Input: part model. Units: mm. Frame: model coordinates. A direction names the side the tool comes from. Coordinates: 2 decimals unless noted, no trailing zeros. Order: outer loops, then holes, each group sorted by start corner. A loop starts at its lowest first (then second) coordinate and runs counter-clockwise, first axis right, second up. Notation, with made-up numbers: (-17, -16) -> (4, -16) arc R20 ccw to (4, 7) -> close; hole circle Ø8 at (29, 52). An arc over 180 degrees is marked (long way). Write each question's results on one line, items separated by ' | '.
```python
from build123d import *

# Parameters (mm, degrees)
F0_W     = 50.8
F0_H     = 19.05
F1_DEPTH = 1123.95
F2_W     = 122.435573
F2_H     = 50.8
F2_W_2   = 93.867282
F2_W_3   = 343.160421
F2_H_2   = 127
F3_DEPTH = 25.4
F4_R     = 0.79375
F5_DEPTH = 25.4
F6_R     = 4.7625
F7_DEPTH = 25.4


with BuildPart() as f1:
    # F0 (on Top) → F1 (new body)
    with BuildSketch(Plane.XY):
        Rectangle(F0_W, F0_H)
    extrude(amount=F1_DEPTH)

    # F2 (on Front) → F3 (cut)
    with BuildSketch(Plane.XZ):
        with Locations((22.446524, 25.4)):
            Rectangle(F2_W, F2_H)
        with Locations((2.720783, 755.65)):
            Rectangle(F2_W_2, F2_H)
        with Locations((-38.781822, 1060.45)):
            Rectangle(F2_W_3, F2_H_2)
    extrude(amount=F3_DEPTH, mode=Mode.SUBTRACT)

    # F4 (on Front) → F5 (cut)
    with BuildSketch(Plane.XZ):
        with Locations((9.525, 101.6)):
            Circle(F4_R)
        with Locations((9.525, 155.575)):
            Circle(F4_R)
        with Locations((9.525, 625.475)):
            Circle(F4_R)
        with Locations((9.525, 679.45)):
            Circle(F4_R)
        with Locations((-9.525, 625.475)):
            Circle(F4_R)
        with Locations((-9.525, 679.45)):
            Circle(F4_R)
        with Locations((-9.525, 101.6)):
            Circle(F4_R)
        with Locations((-9.525, 155.575)):
            Circle(F4_R)
    extrude(amount=-F5_DEPTH, mode=Mode.SUBTRACT)

    # F6 (on Front) → F7 (cut)
    with BuildSketch(Plane.XZ):
        with Locations((15.875, 76.2)):
            Circle(F6_R)
        with Locations((-15.875, 76.2)):
            Circle(F6_R)
        with Locations((-15.875, 304.8)):
            Circle(F6_R)
    extrude(amount=F7_DEPTH, mode=Mode.SUBTRACT)


solid = f1.part
```
(1) Cut plane A-A, the plane y = -6. Count the separate pieces of the cut face and the enclosed holes in it, plus the area to 3 significant figures.
Return value:
separate pieces: 2 | enclosed holes: 3 | area: 45,300 mm2
(2) Pin query (flat end, axial travel): P1, Ø5.5, axis at x = -15.875, z = 76.2, coming from the -Y side; P2, Ø0.5, axis at x = 9.5, z = 101.5, coming from the +Y side. Return the tip coordinate at first contact, or that it passes through.
Return value:
P1: y = 0 | P2: y = 0
(3) Mould query, pull axis Z, two halves, no side actions, for faces 1 (the face through (0, 9.525, 554)), 2 (the face through (0, 0, 756)). Classes: +Z half, -Z half, draft (parallel to the pull), parting line (faces both ways), or undercut.
Return value:
face 1: draft | face 2: undercut
(4) Line query: line 1 along Z through (x, y) = (20, -3); line 2 along X through (y, z) = (-3, 76); line 3 along Z through (x, y) = (9.5, 3.75). Output: solid intervals per line, ascending. Write a range as from..to.
Return value:
line 1: 50.8..73.82, 78.58..730.25, 781.05..996.95 | line 2: -25.4..-20.63, -11.12..11.12, 20.63..25.4 | line 3: 0..100.81, 102.39..154.78, 156.37..624.68, 626.27..678.66, 680.24..1123.95
(5) Cut plane B-B, the plane z = 741.5. Return loops of the section in (x, y) (3 decimals).
Return value:
outline: (-25.4, 0) -> (25.4, 0) -> (25.4, 9.525) -> (-25.4, 9.525) -> close
(6) Reachability of faces 3 (the face through (0, 0, 26)), 4 (the face through (0, 0, 1061)), 5 (the face through (-25.4, 0, 554)) from +Z, -Z, +X, -X, +Y, -Y: full face, straight path, thin tool, end or side. Return the list, or none.
Return value:
face 3: -Z, +X, -X, -Y | face 4: +Z, +X, -X, -Y | face 5: +Z, -Z, -X, +Y, -Y
